from build123d import *

# Parameters (mm, degrees)
ESQUISSE1_R                  = 1.5
BOSS_EXTRU_1_DEPTH           = 1.5
CONG_2_R                     = 1
ESQUISSE2_R                  = 1.5
ENL_V_MAT_EXTRU_1_DEPTH      = 238.959306119
R_P_TITION_CIRCULAIRE1_COUNT = 4
R_P_TITION_CIRCULAIRE1_ANGLE = 60
SYM_TRIE1_COPY_1_SKETCH_R    = 1.5
SYM_TRIE1_COPY_1_DEPTH       = 238.959306119
SYM_TRIE1_COPY_2_SKETCH_R    = 1.5
SYM_TRIE1_COPY_2_DEPTH       = 238.959306119
SYM_TRIE1_COPY_3_SKETCH_R    = 1.5
SYM_TRIE1_COPY_3_DEPTH       = 238.959306119
ENL_V_MAT_EXTRU_2_DEPTH      = 238.959306119
CONG_3_R                     = 1


with BuildPart() as part:
    # Esquisse1 → Boss.-Extru.1 (new body)
    with BuildSketch(Plane(origin=(0, 0, 0), x_dir=(1, 0, 0), z_dir=(0, 1, 0))):
        with BuildLine():
            Line((-130, -60), (130, -60))
            Line((130, -60), (130, -61.5))
            Line((130, -61.5), (162.769008107, -61.5))
            ThreePointArc((162.769008107, -61.5), (98.931794687, -143.138045257), (0, -174))
            ThreePointArc((0, -174), (-98.931794687, -143.138045257), (-162.769008107, -61.5))
            Line((-162.769008107, -61.5), (-130, -61.5))
            Line((-130, -61.5), (-130, -60))
        make_face()
        with Locations(Location((-120, -69, 0), (0, 0, 270))):
            Circle(ESQUISSE1_R, mode=Mode.SUBTRACT)
        with Locations(Location((120, -69, 0), (0, 0, 90))):
            Circle(ESQUISSE1_R, mode=Mode.SUBTRACT)
    extrude(amount=BOSS_EXTRU_1_DEPTH)

    # Congé2
    cong_2_edges = [part.edges().sort_by_distance(p)[0] for p in [
        (-130, 0.75, 60),
        (130, 0.75, 60),
        (162.769008107, 0.75, 61.5),
        (-162.769008107, 0.75, 61.5),
    ]]
    fillet(cong_2_edges, radius=CONG_2_R)

    # Esquisse2 → Enlèv. mat.-Extru.1 (cut, through all)
    with BuildSketch(Plane(origin=(0, 1.5, 0), x_dir=(1, 0, 0), z_dir=(0, 1, 0))):
        with Locations(Location((-15, -167.329017209, 0), (0, 0, 270))):
            Circle(ESQUISSE2_R)
    enl_v_mat_extru_1 = extrude(amount=-ENL_V_MAT_EXTRU_1_DEPTH, mode=Mode.SUBTRACT)

    # Répétition circulaire1: Enlèv. mat.-Extru.1 ×4 about axis
    r_p_tition_circulaire1_axis = Axis((0, 0, 0), (0, -1, 0))
    for i in range(1, R_P_TITION_CIRCULAIRE1_COUNT):
        add(enl_v_mat_extru_1.rotate(r_p_tition_circulaire1_axis, i * R_P_TITION_CIRCULAIRE1_ANGLE / (R_P_TITION_CIRCULAIRE1_COUNT - 1)), mode=Mode.SUBTRACT)

    # Symétrie1: Enlèv. mat.-Extru.1 across plane
    add(enl_v_mat_extru_1.mirror(Plane(origin=(0, 0, 0), x_dir=(0, 0, 1), z_dir=(1, 0, 0))), mode=Mode.SUBTRACT)

    # Symétrie1 copy 1 sketch → Symétrie1 copy 1 (cut, through all)
    with BuildSketch(Plane(origin=(0, 1.5, 0), x_dir=(-0.9396926207859081, 0, 0.3420201433256695), z_dir=(0, 1, 0))):
        with Locations((-15, 167.329017209)):
            Circle(SYM_TRIE1_COPY_1_SKETCH_R)
    extrude(amount=-SYM_TRIE1_COPY_1_DEPTH, mode=Mode.SUBTRACT)

    # Symétrie1 copy 2 sketch → Symétrie1 copy 2 (cut, through all)
    with BuildSketch(Plane(origin=(0, 1.5, 0), x_dir=(-0.766044443118977, 0, 0.6427876096865406), z_dir=(0, 1, 0))):
        with Locations((-15, 167.329017209)):
            Circle(SYM_TRIE1_COPY_2_SKETCH_R)
    extrude(amount=-SYM_TRIE1_COPY_2_DEPTH, mode=Mode.SUBTRACT)

    # Symétrie1 copy 3 sketch → Symétrie1 copy 3 (cut, through all)
    with BuildSketch(Plane(origin=(0, 1.5, 0), x_dir=(-0.4999999999999978, 0, 0.8660254037844399), z_dir=(0, 1, 0))):
        with Locations((-15, 167.329017209)):
            Circle(SYM_TRIE1_COPY_3_SKETCH_R)
    extrude(amount=-SYM_TRIE1_COPY_3_DEPTH, mode=Mode.SUBTRACT)

    # Esquisse3 → Enlèv. mat.-Extru.2 (cut, through all)
    with BuildSketch(Plane(origin=(0, 1.5, 0), x_dir=(1, 0, 0), z_dir=(0, 1, 0))):
        Polygon((-88, -60), (10, -60), (10, -63), (-18, -63), (-18, -72), (-88, -72), align=None)
    extrude(amount=-ENL_V_MAT_EXTRU_2_DEPTH, mode=Mode.SUBTRACT)

    # Congé3
    cong_3_edges = [part.edges().sort_by_distance(p)[0] for p in [
        (-18, 0.75, 72),
        (-88, 0.75, 72),
        (-88, 0.75, 60),
        (10, 0.75, 60),
        (10, 0.75, 63),
        (-18, 0.75, 63),
    ]]
    fillet(cong_3_edges, radius=CONG_3_R)


solid = part.part
Design review of the part built by this model. Coordinates are the model's own, in mm. Coordinates: 2 decimals unless noted, no trailing zeros. Loops run counter-clockwise (first coordinate to the right, second up) from the corner with the lowest first, then second, coordinate; pieces in that order, holes last.
Item 1: Add section B-B (x = 95.5). Write out the cut boundary in (y, z).
Completed:
outline: (0, 60) - (1.5, 60) - (1.5, 145.45) - (0, 145.45) - close
Item 2: Add section A-A (y = 0.9). Give the number of separate pieces and of enclosed holes in the cut face, and give its area (3 significant figures).
Completed:
separate pieces: 1
enclosed holes: 10
area: 26,000 mm2
Item 3: Wall thickness on L1, parallel to X at y = 0.95, z = 151; L2, parallel to X at y = 0.25, z = 68; L3, parallel to X at y = 0.65, z = 128.5: over which ranges is each line inside the solid? List them lowest first.
Completed:
L1: x = -86.46 to -72.34, -70.31 to 70.31, 72.34 to 86.46
L2: x = -160.16 to -121.12, -118.88 to -88, -18 to 118.88, 121.12 to 160.16
L3: x = -117.32 to 117.32
Item 4: Add section C-C (z = 123.5). Write out the cut boundary in (x, y).
Completed:
outline: (-122.57, 0) - (122.57, 0) - (122.57, 1.5) - (-122.57, 1.5) - close
Item 5: Clearance check with flat-ended pins moving along their axes: pin 1 (0.8 mm diameter, centred on x = -143, y = 0.5, fed in from -Z); pin 2 (0.5 mm diameter, centred on y = 1, z = 61.5, fed in from -X); pin 3 (0.8 mm diameter, centred on x = -1, y = 0.5, fed in from -Z). State where each tip first meets the part, or that it passes through.
Completed:
pin 1: stops at z = 61.5
pin 2: stops at x = -161.98
pin 3: stops at z = 63
